The figure shows three views and two pictorial views of one solid part (mm, origin at its lowest corner). Answer the questions. A direction names the side the tool comes from. Coordinates: 2 decimals unless noted, no trailing zeros. Order: outer loops, then holes, each group sorted by start corner. A loop starts at its lowest first (then second) coordinate and runs counter-clockwise, first axis right, second up. Notation, with made-up numbers: (42.5, 58.25) - (67.5, 58.25) arc R26 cw to (67.5, 74.25) - close; hole circle Ø10 at (15, 0.25). An arc over 180 degrees is marked (long way). Use one line per item in the form item = value. Start each with the question number.
Item 1: Section A-A, the plane x = 1.9 is taken. Write down the section's boundary in (y, z).
Item 2: This flat-tipped pin is pushed along its axis until it touches: pin 1 Ø3 at (y, z) = (2.5, 4) entering from -X. Where does it stop, or does it pass through?
Item 3: A tool of negligible diameter and unlimited length cuts with its end or side. For the marked faces 1 and 2, from which of +Z, -Z, +X, -X, +Y, -Y can it reach the whole face along a straight path? Write none if from no direction.
Item 4: Section B-B, the plane z = 5 is taken. Write down the section's boundary in (x, y), and give its area (3 significant figures).
Item 5: Consider line 1 along Y through (x, z) = (3.15, 2.75); line 2 along X through (y, z) = (1.75, 1.75); line 3 along X through (y, z) = (1.45, 4). Determine where each line is inside the solid, lowest interval first. Write a range as [from, to].
Item 6: Section D-D, the plane y = 4.15 is taken. Write down the section's boundary in (x, z), and give its area (3 significant figures).
Item 7: The mould has two halves that part along Y. Classify the marked faces 3, 4 and 5: released by +Y, released by -Y, zero draft, split by the parting line, or undercut.
Item 8: Section C-C, the plane y = 2.2 is taken. Write down the section's boundary in (x, z).
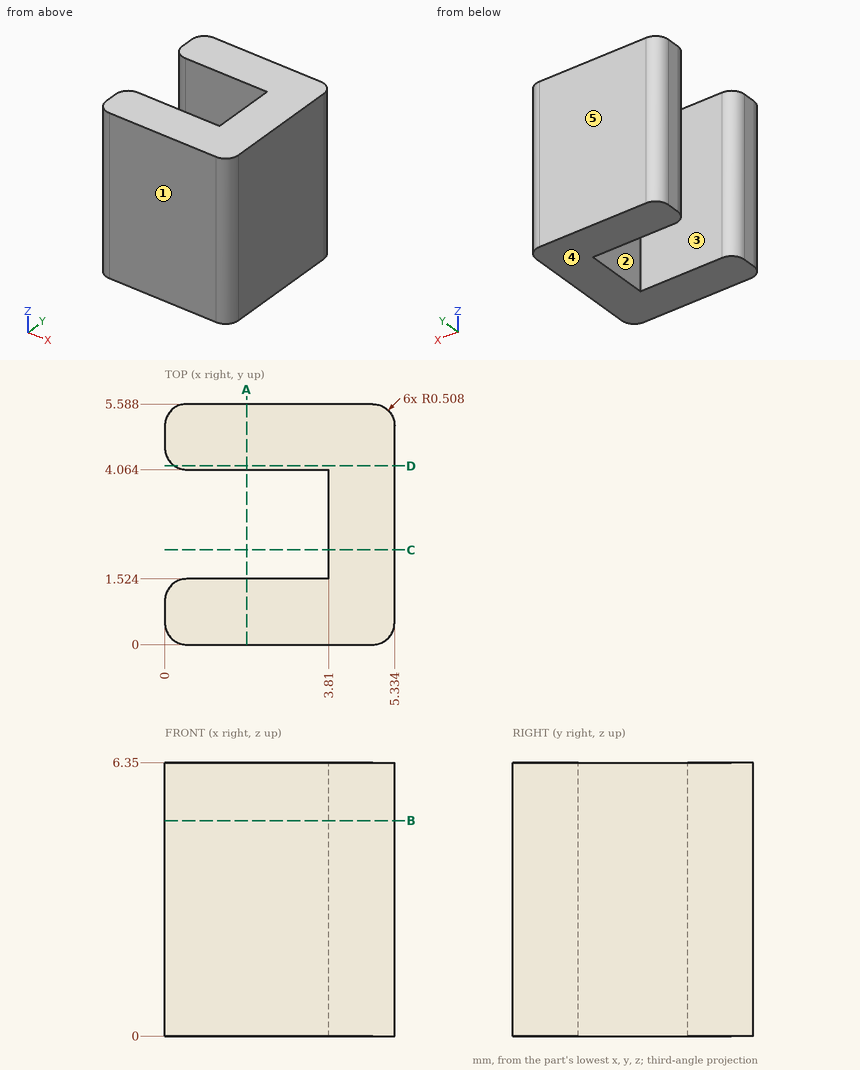
Response:
q1.outline = (0, 0) - (1.52, 0) - (1.52, 6.35) - (0, 6.35) - close; (4.06, 0) - (5.59, 0) - (5.59, 6.35) - (4.06, 6.35) - close
q2.pin_1 = 0
q3.face_1 = +Z, -Z, +X, -X, -Y
q3.face_2 = +Z, -Z, -X
q4.outline = (0, 0.51) arc R0.51 ccw to (0.51, 0) - (4.83, 0) arc R0.51 ccw to (5.33, 0.51) - (5.33, 5.08) arc R0.51 ccw to (4.83, 5.59) - (0.51, 5.59) arc R0.51 ccw to (0, 5.08) - (0, 4.57) arc R0.51 ccw to (0.51, 4.06) - (3.81, 4.06) - (3.81, 1.52) - (0.51, 1.52) arc R0.51 ccw to (0, 1.02) - close
q4.area = 19.8 mm2
q5.line_1 = [0, 1.52], [4.06, 5.59]
q5.line_2 = [3.81, 5.33]
q5.line_3 = [0.24, 5.33]
q6.outline = (0.23, 0) - (5.33, 0) - (5.33, 6.35) - (0.23, 6.35) - close
q6.area = 32.4 mm2
q7.face_3 = undercut
q7.face_4 = zero draft
q7.face_5 = released by +Y
q8.outline = (3.81, 0) - (5.33, 0) - (5.33, 6.35) - (3.81, 6.35) - close
